Can you work these out from the drawing? Everything is in mm from the part's minimum corner. Coordinates: 2 decimals unless noted, no trailing zeros. Order: outer loops, then holes, each group sorted by start corner. A loop starts at its lowest first (then second) coordinate and runs counter-clockwise, first axis right, second up. Notation, with made-up numbers: (74.5, -26) -> (127.5, -26) arc R5 ccw to (127.5, -17) -> close; hole circle Ø7 at (47.25, 2.25). An arc over 180 degrees is marked (long way). Use a Markdown table: item, result. Add a question column.
1) If we section it at C-C (y = 0.85): Give the number of separate pieces and of enclosed holes in the cut face, plus the area to 3 significant figures.
2) If I drill on L1, parallel to Z at x = 47, y = 1.85 (1 decimal); L2, parallel to X at y = 2.4, z = 56; L3, parallel to X at y = 2.8, z = 19.5, over which ranges is the centre line in solid material (lowest first)? Write a range as [from, to].
3) If we section it at B-B (z = 14): Write out the boundary of the cut face in (x, y).
4) Will these pins go through, and if not, where does the flat tip stop? pin 1 Ø15.5 at (x, z) = (39.5, 14) entering from -Y; pin 2 Ø0.9 at (y, z) = (1, 36.5) entering from +X; pin 3 Ø1.5 at (x, y) = (52, 2) entering from -Z; pin 4 Ø1.5 at (y, z) = (1, 8) entering from -X.
5) If we section it at A-A (x = 13.5): Write out the boundary of the cut face in (y, z).
6) If we section it at D-D (z = 52): Write out the boundary of the cut face in (x, y).
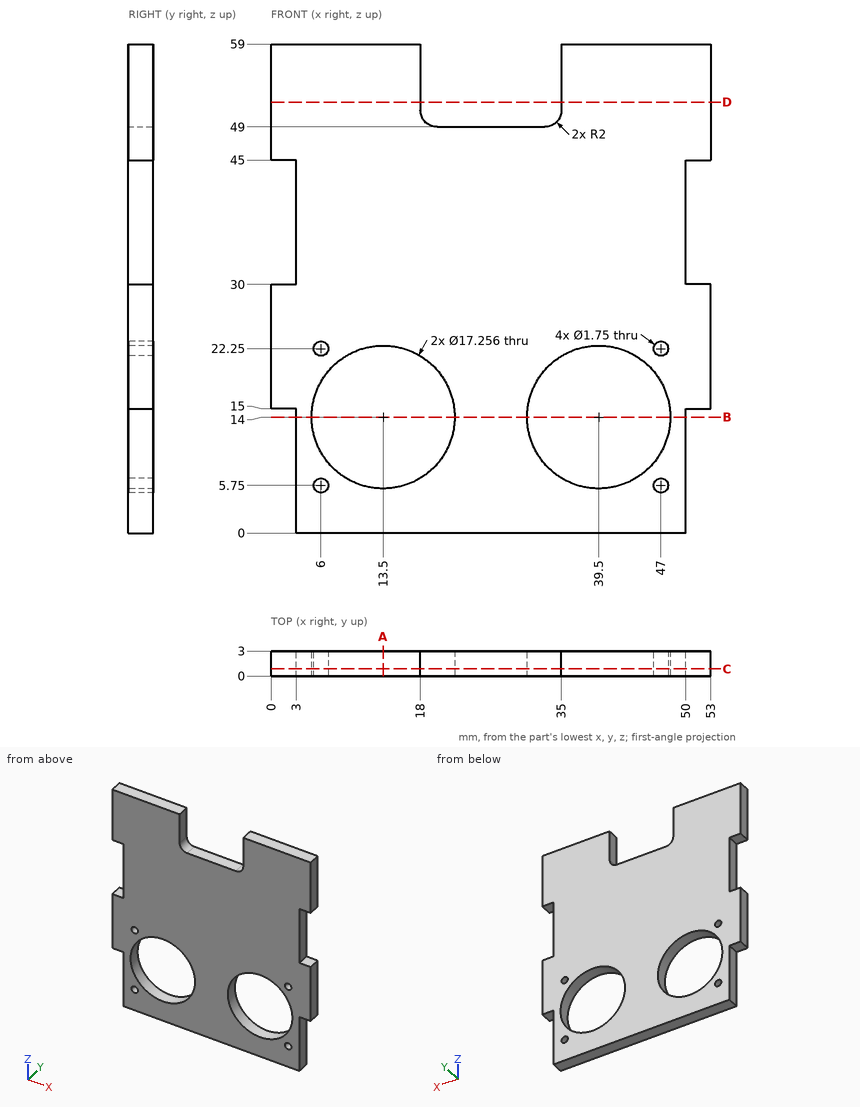
Answer sheet:
| question | item | result |
|---|---|---|
| 1 | separate pieces | 1 |
| 1 | enclosed holes | 6 |
| 1 | area | 2,300 mm2 |
| 2 | L1 | [0, 4.9], [6.6, 9.7], [18.3, 21.4], [23.1, 59] |
| 2 | L2 | [0, 18], [35, 53] |
| 2 | L3 | [0, 6.85], [20.15, 32.85], [46.15, 53] |
| 3 | outline | (3, 0) -> (4.87, 0) -> (4.87, 3) -> (3, 3) -> close; (22.13, 0) -> (30.87, 0) -> (30.87, 3) -> (22.13, 3) -> close; (48.13, 0) -> (50, 0) -> (50, 3) -> (48.13, 3) -> close |
| 4 | pin 1 | through |
| 4 | pin 2 | x = 50 |
| 4 | pin 3 | z = 15 |
| 4 | pin 4 | x = 3 |
| 5 | outline | (0, 0) -> (3, 0) -> (3, 5.37) -> (0, 5.37) -> close; (0, 22.63) -> (3, 22.63) -> (3, 59) -> (0, 59) -> close |
| 6 | outline | (0, 0) -> (18, 0) -> (18, 3) -> (0, 3) -> close; (35, 0) -> (53, 0) -> (53, 3) -> (35, 3) -> close |
